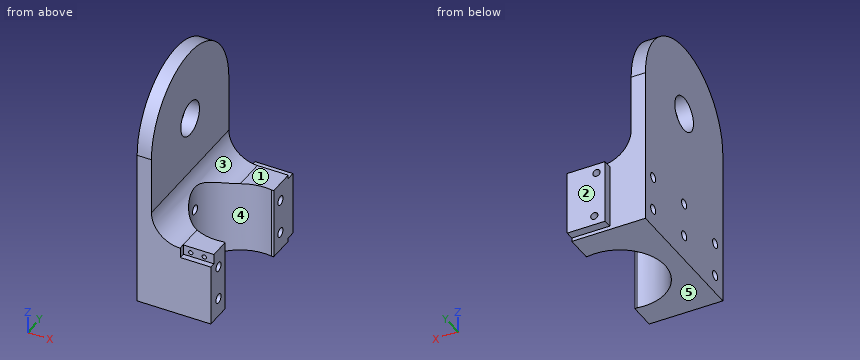
```python
from build123d import *

# Parameters (mm, degrees)
CENTRE_HOLE_FOR_L2_DEPTH      = 40
CENTRE_HOLE_FOR_L2_DEPTH_BACK = 10
SKETCH1_R                     = 39.1
SKETCH1_R_2                   = 31.75
MAIN_STRUCTURE_DEPTH          = 60
MAIN_STRUCTURE_DEPTH_BACK     = 50
SKETCH2_W                     = 90
SKETCH2_H                     = 100
SKETCH2_R                     = 31.75
BEARING_CURVE_DEPTH           = 10
SKETCH6_R                     = 10.5
SHAFT_HOLE_DEPTH              = 10
WRIST_CUTOUT_DEPTH            = 186.809041761
SURFACECUT1_START             = 5
SURFACECUT1_OUTLINE_R         = 10.5
SURFACECUT1_DEPTH             = 40
SKETCH11_W                    = 25
SKETCH11_H                    = 45
SKETCH11_R                    = 2.525
BOSS_EXTRUDE1_DEPTH           = 6
SKETCH15_W                    = 19.8
SKETCH15_H                    = 7
CUT_EXTRUDE4_DEPTH            = 4
CUT_EXTRUDE5_REACH            = 188.893
CUT_EXTRUDE5_END_RADIUS       = 31.75
SKETCH16_R                    = 1.5
CUT_EXTRUDE6_DEPTH            = 168.7378908
CUT_EXTRUDE6_DEPTH_BACK       = 168.7378908
SKETCH18_R                    = 3.25
SKETCH19_R                    = 3.25
CUT_EXTRUDE7_DEPTH            = 168.7378908
SKETCH9_R                     = 12.05
CUT_EXTRUDE8_DEPTH            = 10
SKETCH20_R                    = 3.25
SKETCH20_W                    = 45
SKETCH20_H                    = 6
BOSS_EXTRUDE2_DEPTH           = 1.5875


# Read off the part's stored shape, not the designer's step: SurfaceCut1
with BuildPart() as part:
    # Sketch1 → Centre Hole for L2 (new, two sides: drawn at the far end of the back side and taken through both)
    with BuildSketch(Plane.XY.offset(-CENTRE_HOLE_FOR_L2_DEPTH_BACK)):
        Circle(SKETCH1_R)
        Circle(SKETCH1_R_2, mode=Mode.SUBTRACT)
    extrude(amount=CENTRE_HOLE_FOR_L2_DEPTH + CENTRE_HOLE_FOR_L2_DEPTH_BACK)


with BuildPart() as body_2:
    # Sketch2 → Main Structure (new, two sides: drawn at the far end of the back side and taken through both)
    with BuildSketch(Plane.XY.offset(40).offset(-MAIN_STRUCTURE_DEPTH_BACK)):
        Rectangle(SKETCH2_W, SKETCH2_H)
        Circle(SKETCH2_R, mode=Mode.SUBTRACT)
    extrude(amount=MAIN_STRUCTURE_DEPTH + MAIN_STRUCTURE_DEPTH_BACK)

    # Sketch3 → Bearing Curve (add)
    with BuildSketch(Plane.ZY.offset(45)):
        with BuildLine():
            Line((100, 50), (100, -50))
            ThreePointArc((100, -50), (150, 0), (100, 50))
        make_face()
    bearing_curve = extrude(amount=-BEARING_CURVE_DEPTH)

    # Upright Mirror: Bearing Curve across plane
    add(bearing_curve.mirror(Plane(origin=(0, 0, 0), x_dir=(0, 0, 1), z_dir=(1, 0, 0))))

    # Sketch6 → Shaft Hole (cut)
    with BuildSketch(Plane.ZY.offset(45)):
        with Locations((100, 0)):
            Circle(SKETCH6_R)
    shaft_hole = extrude(amount=-SHAFT_HOLE_DEPTH, mode=Mode.SUBTRACT)

    # Sketch4 → Wrist Cutout (cut, through all)
    with BuildSketch(Plane(origin=(0, 50, 0), x_dir=(1, 0, 0), z_dir=(0, 1, 0))):
        with BuildLine():
            Line((-35, -100), (-35, -60))
            ThreePointArc((-35, -60), (-29.142135624, -45.857864376), (-15, -40))
            Line((-15, -40), (15, -40))
            ThreePointArc((15, -40), (29.142135624, -45.857864376), (35, -60))
            Line((35, -60), (35, -100))
            Line((35, -100), (-35, -100))
        make_face()
    extrude(amount=-WRIST_CUTOUT_DEPTH, mode=Mode.SUBTRACT)

    # Bearing Mirror: Shaft Hole across plane
    add(shaft_hole.mirror(Plane(origin=(0, 0, 0), x_dir=(0, 0, 1), z_dir=(1, 0, 0))), mode=Mode.SUBTRACT)


with BuildPart() as surfacecut1_tool:
    # SurfaceCut1 outline → SurfaceCut1 (new body)
    with BuildSketch(Plane.YZ.offset(SURFACECUT1_START)):
        with BuildLine():
            ThreePointArc((50, 100), (0, 150), (-50, 100))
            Line((-50, 100), (-50, -10))
            Line((-50, -10), (50, -10))
            Line((50, -10), (50, 100))
        make_face()
        with Locations((0, 100)):
            Circle(SURFACECUT1_OUTLINE_R, mode=Mode.SUBTRACT)
    extrude(amount=SURFACECUT1_DEPTH)


with BuildPart() as part_1:
    add(part.part)

    # SurfaceCut1: cut by surfacecut1_tool
    add(surfacecut1_tool.part, mode=Mode.SUBTRACT)


with BuildPart() as body_2_1:
    add(body_2.part)

    # SurfaceCut1: cut by surfacecut1_tool
    add(surfacecut1_tool.part, mode=Mode.SUBTRACT)

    # Sketch15 → Cut-Extrude4 (cut)
    with BuildSketch(Plane(origin=(0, -50, 0), x_dir=(-1, 0, 0), z_dir=(0, -1, 0))):
        with Locations((4.9, -36.5)):
            Rectangle(SKETCH15_W, SKETCH15_H)
    extrude(amount=-CUT_EXTRUDE4_DEPTH, mode=Mode.SUBTRACT)


with BuildPart() as body_3:
    # Sketch11 → Boss-Extrude1 (new body)
    with BuildSketch(Plane(origin=(0, 50, 0), x_dir=(1, 0, 0), z_dir=(0, 1, 0))):
        with Locations((-7.5, -15)):
            Rectangle(SKETCH11_W, SKETCH11_H)
        with Locations(Location((-12.4125, 1, 0), (0, 0, 270))):
            Circle(SKETCH11_R, mode=Mode.SUBTRACT)
        with Locations(Location((-14, -31, 0), (0, 0, 270))):
            Circle(SKETCH11_R, mode=Mode.SUBTRACT)
    extrude(amount=BOSS_EXTRUDE1_DEPTH)


with BuildPart() as cut_extrude5_tool:
    # Cut-Extrude5: up to this cylinder (the profile starts outside it)
    cut_extrude5_end = Plane(origin=(0, 0, 35.9), z_dir=(0, 0, 1)) * Cylinder(CUT_EXTRUDE5_END_RADIUS, 442.286, mode=Mode.PRIVATE)
    # Sketch16 → Cut-Extrude5 (new, up to the surface)
    with BuildSketch(Plane(origin=(0, -46, 0), x_dir=(-1, 0, 0), z_dir=(0, -1, 0)), mode=Mode.PRIVATE) as cut_extrude5_sk1:
        with Locations(Location((9.65, -35.9, 0), (0, 0, 90))):
            Circle(SKETCH16_R)
    cut_extrude5_tool1 = extrude(cut_extrude5_sk1.sketch, amount=-CUT_EXTRUDE5_REACH, mode=Mode.PRIVATE) - cut_extrude5_end
    add(cut_extrude5_tool1.solids().sort_by_distance((-9.65, -46, 35.9))[0])
    # Sketch16 → Cut-Extrude5 (new, up to the surface)
    with BuildSketch(Plane(origin=(0, -46, 0), x_dir=(-1, 0, 0), z_dir=(0, -1, 0)), mode=Mode.PRIVATE) as cut_extrude5_sk2:
        with Locations(Location((0.15, -35.9, 0), (0, 0, 90))):
            Circle(SKETCH16_R)
    cut_extrude5_tool2 = extrude(cut_extrude5_sk2.sketch, amount=-CUT_EXTRUDE5_REACH, mode=Mode.PRIVATE) - cut_extrude5_end
    add(cut_extrude5_tool2.solids().sort_by_distance((-0.15, -46, 35.9))[0])


with BuildPart() as part_2:
    add(part_1.part)

    # Cut-Extrude5: cut by cut_extrude5_tool
    add(cut_extrude5_tool.part, mode=Mode.SUBTRACT)


with BuildPart() as body_2_2:
    add(body_2_1.part)

    # Cut-Extrude5: cut by cut_extrude5_tool
    add(cut_extrude5_tool.part, mode=Mode.SUBTRACT)


with BuildPart() as cut_extrude6_tool:
    # Sketch18 → Cut-Extrude6 (new, two sides: drawn at the far end of the back side and taken through both)
    with BuildSketch(Plane.ZY.offset(45).offset(-CUT_EXTRUDE6_DEPTH_BACK)):
        with Locations((8, 0)):
            Circle(SKETCH18_R)
        with Locations((32, 0)):
            Circle(SKETCH18_R)
    extrude(amount=CUT_EXTRUDE6_DEPTH + CUT_EXTRUDE6_DEPTH_BACK)


with BuildPart() as part_3:
    add(part_2.part)

    # Cut-Extrude6: cut by cut_extrude6_tool
    add(cut_extrude6_tool.part, mode=Mode.SUBTRACT)


with BuildPart() as body_2_3:
    add(body_2_2.part)

    # Cut-Extrude6: cut by cut_extrude6_tool
    add(cut_extrude6_tool.part, mode=Mode.SUBTRACT)


with BuildPart() as cut_extrude7_tool:
    # Sketch19 → Cut-Extrude7 (new, through all)
    with BuildSketch(Plane.ZY.offset(45)):
        with Locations((32, 0)):
            Circle(SKETCH19_R)
        with Locations((8, 0)):
            Circle(SKETCH19_R)
        with Locations((3, 40)):
            Circle(SKETCH19_R)
        with Locations((27, 40)):
            Circle(SKETCH19_R)
        with Locations((3, -40)):
            Circle(SKETCH19_R)
        with Locations((27, -40)):
            Circle(SKETCH19_R)
    extrude(amount=-CUT_EXTRUDE7_DEPTH)


with BuildPart() as part_4:
    add(part_3.part)

    # Cut-Extrude7: cut by cut_extrude7_tool
    add(cut_extrude7_tool.part, mode=Mode.SUBTRACT)



with BuildPart() as body_2_4:
    add(body_2_3.part)

    # Cut-Extrude7: cut by cut_extrude7_tool
    add(cut_extrude7_tool.part, mode=Mode.SUBTRACT)

    # Sketch9 → Cut-Extrude8 (cut)
    with BuildSketch(Plane(origin=(-35, 0, 0), x_dir=(0, 0, -1), z_dir=(1, 0, 0))):
        with Locations((-100, 0)):
            Circle(SKETCH9_R)
    extrude(amount=-CUT_EXTRUDE8_DEPTH, mode=Mode.SUBTRACT)


with BuildPart() as part_5:
    add(part_4.part)

    add(body_2_4.part)  # Boss-Extrude2 merges body 2

    add(body_3.part)  # Boss-Extrude2 merges body 3
    # Sketch20 → Boss-Extrude2 (add)
    # profile 1 of 3: a face of its own
    with BuildSketch(Plane(origin=(5, 0, 0), x_dir=(0, 0, -1), z_dir=(1, 0, 0))):
        Polygon((-40, 50), (-40, 38.778989157), (-40, 31.353827518), (10, 31.353827518), (10, 38.778989157), (10, 50), (7.5, 50), (-37.5, 50), align=None)
        with Locations(Location((-27, 40, 0), (0, 0, 180))):
            Circle(SKETCH20_R, mode=Mode.SUBTRACT)
        with Locations(Location((-3, 40, 0), (0, 0, 180))):
            Circle(SKETCH20_R, mode=Mode.SUBTRACT)
    # profile 2 of 3: a face of its own
    with BuildSketch(Plane(origin=(5, 0, 0), x_dir=(0, 0, -1), z_dir=(1, 0, 0))):
        with Locations((-15, 53)):
            Rectangle(SKETCH20_W, SKETCH20_H)
    # profile 3 of 3: a face of its own
    with BuildSketch(Plane(origin=(5, 0, 0), x_dir=(0, 0, -1), z_dir=(1, 0, 0))):
        Polygon((10, -50), (10, -38.778989157), (10, -31.353827518), (-40, -31.353827518), (-40, -38.778989157), (-40, -46), (-33, -46), (-33, -50), align=None)
        with Locations(Location((-27, -40, 0), (0, 0, 180))):
            Circle(SKETCH20_R, mode=Mode.SUBTRACT)
        with Locations(Location((-3, -40, 0), (0, 0, 180))):
            Circle(SKETCH20_R, mode=Mode.SUBTRACT)
    extrude(amount=BOSS_EXTRUDE2_DEPTH)


solid = part_5.part
```
The model under review builds one solid part; all positions refer to its coordinate system, in mm. Face numbers are marked on the shaded views. A direction names the side the tool comes from. Give positions to 0.01 mm unless a question says otherwise; leave off trailing zeros. Write each loop counter-clockwise with the first axis right and the second up, starting at its lowest first coordinate (ties: lowest second). Pieces come first, ordered by that corner, then holes. Notation, with made-up numbers: M 48.5,-21.5 L 66.5,-21.5 A30 ccw 66.5,8.5 Z; hole C -14.5,-23.75 d6. An arc over 180 degrees is marked long. Write each question's results on one line, items separated by ' | '. Start each with the question number.
1. We need section B-B (x = -26.5). Write out the cut boundary in (y, z), and give its area (4 significant figures).
2. We need section A-A (y = 40). Write out the cut boundary in (x, z), and give its area (3 significant figures).
3. For the marked faces 1 and 2, list the 3-axis set-ups (+Z, -Z, +X, -X, +Y, -Y) from which the entire face can be reached by the end or side of a thin tool; tool diameter is ignored.
4. For probe 1 along X at (y, z) = (-44, 35.9); probe 2 along Z at (x, y) = (-15, 40); probe 3 along Z at (x, y) = (-9.65, -40.5), list the stretches that pass through material, from the lowest coordinate up. Write a range as [from, to].
5. Mouldability with a two-part tool opening along X and no side actions: class the marked faces 3, 4 and 5 as released by +X, released by -X, zero draft, split by the parting line, or undercut.
6. We need section D-D (y = 5). Write out the cut boundary in (x, z).
7. We need section C-C (x = -3.5). Write out the cut boundary in (y, z).
8. Insertion check: pin 1 Ø6 at (y, z) = (36.5, 75.5) entering from +X; pin 2 Ø4 at (x, z) = (-9.65, 35.9) entering from -Y; pin 3 Ø1 at (x, y) = (-38.5, -1) entering from +Z. Each pin has a flat end and moves straight along its axis. Give the tip position at first contact, or say it passes through.
Results found:
1) outline: M -50,-10 L -17.49,-10 L -17.49,43.64 L -50,43.64 Z; M 17.49,-10 L 50,-10 L 50,43.64 L 17.49,43.64 Z; hole C -40,3 d6.5; hole C -40,27 d6.5; hole C 40,3 d6.5; hole C 40,27 d6.5 | area: 3,355 mm^2
2) outline: M -45,-10 L 6.59,-10 L 6.59,-0.25 L -45,-0.25 Z; M -45,6.25 L 6.59,6.25 L 6.59,23.75 L -45,23.75 Z; M -45,30.25 L 6.59,30.25 L 6.59,40 L -15,40 A20 cw -35,60 L -35,130 L -45,130 Z | area: 2,890 mm^2
3) face 1: +Z, +X, +Y, -Y | face 2: +Z, -Z, +X, -X, +Y
4) probe 1: x = [-45, -11.15], [-8.15, -1.65], [1.35, 6.59] | probe 2: z = [-10, -0.25], [6.25, 23.75], [30.25, 40] | probe 3: z = [-10, -0.21], [6.21, 23.79], [30.21, 34.4], [37.4, 40]
5) face 3: released by +X | face 4: undercut | face 5: zero draft
6) outline: M -45,-10 L -31.35,-10 L -31.35,48.49 A20 cw -35,60 L -35,89.04 L -45,89.04 Z; M -45,110.96 L -35,110.96 L -35,149.75 L -45,149.75 Z
7) outline: M -50,-10 L -31.56,-10 L -31.56,40 L -46,40 L -46,33 L -50,33 Z; M 31.56,-10 L 50,-10 L 50,-7.5 L 56,-7.5 L 56,37.5 L 50,37.5 L 50,40 L 31.56,40 Z; hole C -40,3 d6.5; hole C -40,27 d6.5; hole C 40,3 d6.5; hole C 40,27 d6.5
8) pin 1: stops at x = -35 | pin 2: stops at y = -46 | pin 3: stops at z = 150
